CAD build for the part. Positions are in the model's coordinates, mm. A direction names the side the tool comes from. Give positions to 0.01 mm unless a question says otherwise; leave off trailing zeros. Loops run counter-clockwise (first coordinate to the right, second up) from the corner with the lowest first, then second, coordinate; pieces in that order, holes last.
Autodesk Inventor part; units mm, degrees
ref_plane "YZ Plane" through (0, 0, 0) normal (1, 0, 0) x (0, 1, 0)
ref_plane "XZ Plane" through (0, 0, 0) normal (0, 1, 0) x (-1, 0, 0)
ref_plane "XY Plane" through (0, 0, 0) normal (0, 0, 1) x (1, 0, 0)
sketch "Sketch1" plane through (0, 0, 0) normal (0, 0, 1) x (1, 0, 0)
  line L0 (45, -50) -> (41, -50) construction
  line L1 (-45, -50) -> (-45, 50) construction
  line L2 (-45, 50) -> (-25, 50)
  line L3 (45, 50) -> (45, 20) construction
  line L4 (45, -50) -> (-45, 50) construction
  line L5 (-45, -50) -> (45, 50) construction
  line L6 (-25, 50) -> (25, 50) construction
  line L7 (25, 50) -> (25, 54)
  line L8 (25, 54) -> (-25, 54)
  line L9 (-25, 54) -> (-25, 50)
  line L10 (-25, -50) -> (25, -50) construction
  line L11 (25, -50) -> (25, -54)
  line L12 (25, -54) -> (-25, -54)
  line L13 (-25, -54) -> (-25, -50)
  line L14 (-45, 50) -> (-49, 50)
  line L15 (-49, 50) -> (-49, 25)
  line L16 (-49, 25) -> (-45, 25)
  line L17 (-45, 25) -> (-45, 50) construction
  line L18 (-45, 0) -> (-45, 25)
  line L19 (-45, 25) -> (-49, 25)
  line L20 (-49, 25) -> (-49, 0) construction
  line L21 (-49, 0) -> (-45, 0)
  line L22 (-45, -25) -> (-45, 0) construction
  line L23 (-45, 0) -> (-49, 0)
  line L24 (-49, 0) -> (-49, -25)
  line L25 (-49, -25) -> (-45, -25)
  line L26 (-45, -50) -> (-45, -25)
  line L27 (-45, -25) -> (-49, -25)
  line L28 (-49, -25) -> (-49, -50) construction
  line L29 (-49, -50) -> (-45, -50) construction
  line L30 (0, -75.6) -> (0, 75.6) construction
  line L31 (45, 20) -> (49, 20)
  line L32 (49, 20) -> (49, -20)
  line L33 (49, -20) -> (45, -20)
  line L34 (45, -20) -> (45, 20) construction
  line L35 (25, 50) -> (41, 50)
  line L36 (-25, 50) -> (25, 50) construction
  line L37 (-25, -50) -> (-45, -50)
  line L38 (25, -50) -> (-25, -50) construction
  line L39 (-68.6, 0) -> (68.6, 0) construction
  line L40 (41, 50) -> (41, 20)
  line L41 (41, 20) -> (45, 20)
  line L42 (45, -20) -> (41, -20)
  line L43 (41, -20) -> (41, -50)
  line L44 (41, 50) -> (45, 50) construction
  line L45 (45, 20) -> (45, -20) construction
  line L46 (45, -20) -> (45, -50) construction
  line L47 (41, -50) -> (25, -50)
  point P0 (0, 0)
  point P1 (41, 35)
  dimension "d0" = 90
  dimension "d1" = 100
  dimension "d2" = 50
  dimension "d3" = 4
  dimension "d4" = 50
  dimension "d5" = 4
  dimension "d6" = 4
  dimension "d7" = 25
  dimension "d10" = 25
  dimension "d17" = 4
  dimension "d18" = 40
  dimension "d20" = 4
extrude "Extrusion1" add sketch "Sketch1" along normal blind 4
properties part number "CarSide_V2" material "Wood (Oak)"
1. Saw through at B-B, the plane y = 44. List the corners of the cut face in (x, z).
Responses:
outline: (-49, 0) - (41, 0) - (41, 4) - (-49, 4) - close
2. Tool access for faces 1 (the face through (-45, 12, 2)), 2 (the face through (-47, -25, 2)), 3 (the face through (25, -52, 2)): list every direction of +Z, -Z, +X, -X, +Y, -Y with a clear straight run to the whole face (end or side of a thin tool).
Responses:
face 1: +Z, -Z, -X
face 2: +Z, -Z, -X, -Y
face 3: +Z, -Z, +X, -Y
3. Saw through at C-C, the plane x = -33. List the corners of the cut face in (y, z), and give its area (3 significant figures).
Responses:
outline: (-50, 0) - (50, 0) - (50, 4) - (-50, 4) - close
area: 400 mm2
4. Drop flat-ended pins along their axis: pin 1 (2 mm diameter, centred on y = -33.5, z = 1, fed in from +X); pin 2 (1.2 mm diameter, centred on x = -47.5, z = 2.5, fed in from -Y); pin 3 (1.2 mm diameter, centred on y = -52.5, z = 1.5, fed in from +X). Give the stop position or say it passes through.
Responses:
pin 1: stops at x = 41
pin 2: stops at y = -25
pin 3: stops at x = 25
5. Saw through at A-A, the plane z = 1.1. List the corners of the cut face in (x, y), and give its area (3 significant figures).
Responses:
outline: (-49, -25) - (-45, -25) - (-45, -50) - (-25, -50) - (-25, -54) - (25, -54) - (25, -50) - (41, -50) - (41, -20) - (49, -20) - (49, 20) - (41, 20) - (41, 50) - (25, 50) - (25, 54) - (-25, 54) - (-25, 50) - (-49, 50) - (-49, 25) - (-45, 25) - (-45, 0) - (-49, 0) - close
area: 9,520 mm2
6. Probe line 1 along X through (y, z) = (6, 3.25); line 2 along Y through (x, z) = (42, 0.35); line 3 along Y through (x, z) = (-32, 1.85). List the from-to ranges inside material, lowest first.
Responses:
line 1: x = -45 to 49
line 2: y = -20 to 20
line 3: y = -50 to 50
7. Pull direction Y, two halves, no side cores. Call faces 4 (the face through (-35, -50, 2)), 5 (the face through (-47, 0, 2)), 6 (the face through (49, 0, 2)): released by +Y, released by -Y, zero draft, split by the parting line, or undercut.
Responses:
face 4: released by -Y
face 5: undercut
face 6: zero draft
